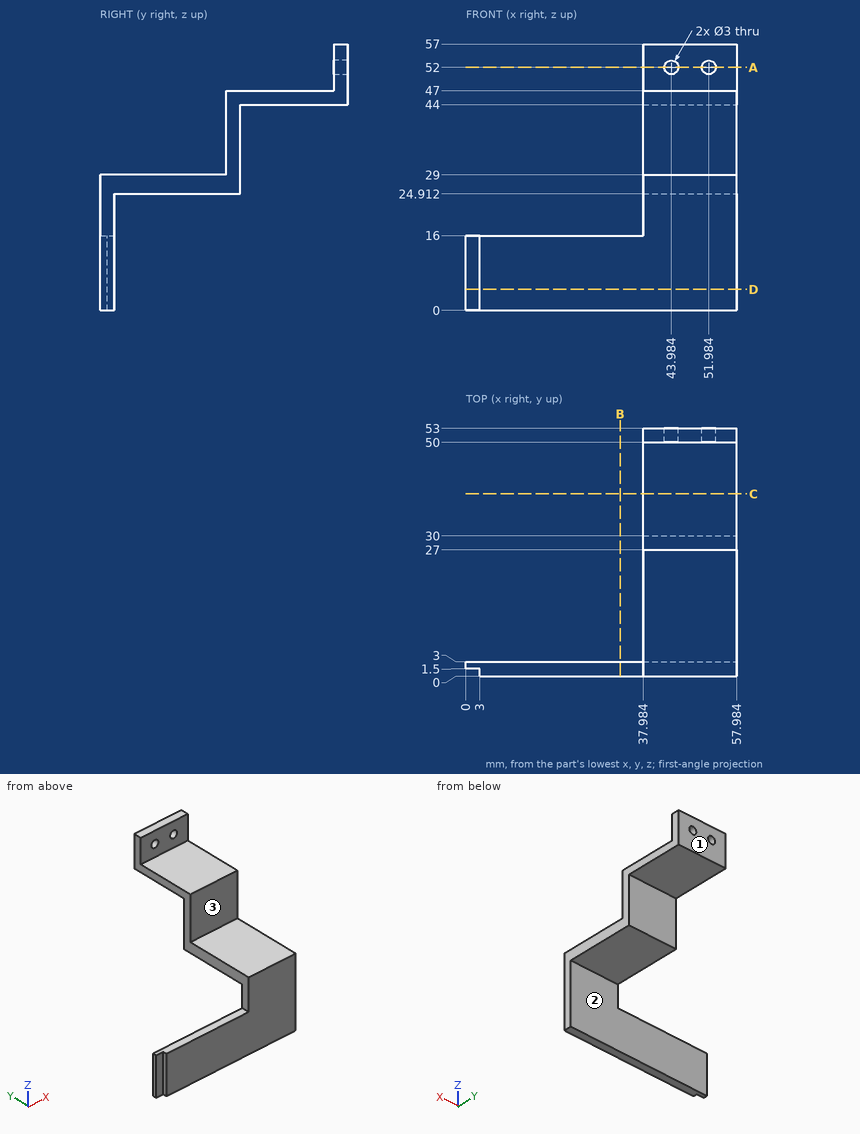
Study the drawing (mm; zero at the part's minimum x, y, z) and answer. A direction names the side the tool comes from. Round coordinates to 2 decimals unless told otherwise and drop trailing zeros. Write each loop counter-clockwise with the first axis right and the second up, starting at its lowest first coordinate (ties: lowest second). Pieces come first, ordered by that corner, then holes.
1) A cutting plane is placed at A-A on z = 52. Determine the outline of the cut face in (x, y).
2) Flat-ended cylindrical pins translate along their axes: P1, Ø2.5, axis at x = 18, y = 1.5, coming from the +Z side; P2, Ø3, axis at x = 50.5, y = 11.5, coming from the -Z side; P3, Ø0.9, axis at x = 2, z = 5, coming from the -Y side. Find the tip coordinate at first contact, or state that the pin passes through.
3) Which of the six approach directions +Z, -Z, +X, -X, +Y, -Y give full straight-line access (tool end or side, diameter ignored) to the marked faces 1, 2 and 3?
4) A cutting plane is placed at C-C on y = 39. Determine the outline of the cut face in (x, z).
5) A cutting plane is placed at B-B on x = 33. Determine the outline of the cut face in (y, z), and give its area (3 significant figures).
6) Consider probe 1 along X at (y, z) = (52, 52); probe 2 along Z at (x, y) = (55, 8); probe 3 along X at (y, z) = (50.5, 47.5). Determine where each line is inside the solid, lowest interval first.
7) A cutting plane is placed at D-D on z = 4.5. Determine the outline of the cut face in (x, y).
Entries:
1. outline: (37.98, 50) - (42.48, 50) - (42.48, 53) - (37.98, 53) - close; (45.48, 50) - (50.48, 50) - (50.48, 53) - (45.48, 53) - close; (53.48, 50) - (57.98, 50) - (57.98, 53) - (53.48, 53) - close
2. P1: stops at z = 16
2. P2: stops at z = 24.91
2. P3: stops at y = 1.5
3. face 1: +Z, -Z, +X, -X, +Y
3. face 2: -Z, +X, -X, +Y
3. face 3: +Z, +X, -X, -Y
4. outline: (37.98, 44) - (57.98, 44) - (57.98, 47) - (37.98, 47) - close
5. outline: (0, 0) - (3, 0) - (3, 16) - (0, 16) - close
5. area: 48.0 mm2
6. probe 1: x = 37.98 to 42.48, 45.48 to 50.48, 53.48 to 57.98
6. probe 2: z = 24.91 to 29
6. probe 3: x = 37.98 to 57.98
7. outline: (0, 1.5) - (3, 1.5) - (3, 0) - (57.98, 0) - (57.98, 3) - (0, 3) - close
